For this review, take the finished solid that the model builds, in its own axes (mm). A direction names the side the tool comes from. Give positions to 0.01 mm unless a question says otherwise; leave off trailing zeros. Order: outer loops, then holes, each group sorted by start corner. A loop starts at its lowest first (then second) coordinate and runs counter-clockwise, first axis right, second up. Notation, with made-up numbers: (-18, 79.5) -> (-4, 79.5) arc R32 ccw to (-4, 107.5) -> close; hole circle Ø10 at (25, 17). An arc over 180 degrees is marked (long way). Use CSV: the item, a comma, the result in double quotes. Start each with the question number.
```python
from build123d import *

# Parameters (mm, degrees)
F0_R     = 4.699
F1_DEPTH = 88.9
F2_R     = 6.35
F2_R_2   = 4.699
F3_DEPTH = 12.7
F4_DEPTH = 2.54


with BuildPart() as f1:
    # F0 (on Front) → F1 (new body)
    with BuildSketch(Plane.XZ):
        Circle(F0_R)
    extrude(amount=F1_DEPTH)

    # F2 (on face) → F3 (join)
    with BuildSketch(Plane.XZ.offset(88.9)):
        Circle(F2_R)
        Circle(F2_R_2, mode=Mode.SUBTRACT)
    extrude(amount=F3_DEPTH)

    # F4 (add): a face of the model
    f4_faces = [f1.faces().sort_by_distance(p)[0] for p in [
        (-6.1703948776, -88.9, 0),
    ]]
    extrude(f4_faces, amount=F4_DEPTH)


solid = f1.part
```
1. Draft analysis for pull direction X (two halves, no side actions). For faces 1 (the face through (-0.61, -42.58, 4.66)), 2 (the face through (0, -86.36, 5)), 3 (the face through (-0.61, -95.16, 4.66)), state which applies: +X half, -X half, draft (parallel to the pull), parting line (faces both ways), or undercut.
2. To check wall thickness, follow L1, parallel to Z at x = 0, y = -95; L2, parallel to Y at x = -4.75, z = -3.25; L3, parallel to Y at x = -1, z = 3. State the ranges of each line that lie inside material, in increasing order. Write a range as [from, to].
3. Consider section C-C (y = -73). State the section outline as (x, z) points, plus the area to 3 significant figures.
4. For faces 4 (the face through (0, -88.9, 0)), 5 (the face through (-1.38, -94.09, -6.2)), list the 3-axis set-ups (+Z, -Z, +X, -X, +Y, -Y) from which the entire face can be reached by the end or side of a thin tool; tool diameter is ignored.
5. Consider section A-A (z = 0). State the section outline as (x, y) points.
6. Consider section B-B (x = 0). State the section outline as (y, z) points.
7. Clearance check with flat-ended pins moving along their axes: P1, Ø2, axis at x = 4, y = -30, coming from the +Z side; P2, Ø4, axis at y = -67.5, z = 0, coming from the +X side; P3, Ø5, axis at x = 4, y = -26, coming from the -Z side; P4, Ø4.5, axis at x = 2.5, z = 1, coming from the -Y side. State where each tip first meets the part, or that it passes through.
Answer list:
1,face 1,"parting line"
1,face 2,"draft"
1,face 3,"undercut"
2,L1,"[-6.35, -4.7], [4.7, 6.35]"
2,L2,"[-101.6, -86.36]"
2,L3,"[-88.9, 0]"
3,outline,"circle Ø9.4 at (0, 0)"
3,area,"69.4 mm2"
4,face 4,"-Y"
4,face 5,"+Y, -Y"
5,outline,"(-6.35, -101.6) -> (-4.7, -101.6) -> (-4.7, -88.9) -> (4.7, -88.9) -> (4.7, -101.6) -> (6.35, -101.6) -> (6.35, -86.36) -> (4.7, -86.36) -> (4.7, 0) -> (-4.7, 0) -> (-4.7, -86.36) -> (-6.35, -86.36) -> close"
6,outline,"(-101.6, -6.35) -> (-86.36, -6.35) -> (-86.36, -4.7) -> (0, -4.7) -> (0, 4.7) -> (-86.36, 4.7) -> (-86.36, 6.35) -> (-101.6, 6.35) -> (-101.6, 4.7) -> (-88.9, 4.7) -> (-88.9, -4.7) -> (-101.6, -4.7) -> close"
7,P1,"z = 3.62"
7,P2,"x = 4.7"
7,P3,"z = -4.45"
7,P4,"y = -101.6"
